The figure shows three views and two pictorial views of one solid part (mm, origin at its lowest corner). Answer the questions. Coordinates: 2 decimals unless noted, no trailing zeros. Loops run counter-clockwise (first coordinate to the right, second up) from the corner with the lowest first, then second, coordinate; pieces in that order, holes last. Notation, with made-up numbers: M 32.5,-3 L 85.5,-3 A14 ccw 85.5,11 Z; hole C -32,35.5 d8. An arc over 180 degrees is marked long. Return JSON: item names as keys, results as strings. Group by question number.
1. Given P1, Ø0.5, axis at x = 36.5, y = 36.5, coming from the +Z side; P2, Ø2.5, axis at x = 1, z = 16, coming from the -Y side; P3, Ø1.1, axis at x = 36, y = 36.5, coming from the -Z side; P4, Ø2.5, axis at x = 1, z = 16.5, coming from the -Y side, each flat-ended and moving along its own axis, determine where each tip first touches the part or whether it passes through.
2. Section B-B (z = 16.5) is taken. Write down the section's boundary in (x, y), then the cut area to 3 significant figures.
3. Section A-A (x = 19.25) is taken. Write down the section's boundary in (y, z), then the cut area to 3 significant figures.
4. Straight lines are drawn through the part: L1, parallel to Z at x = 1, y = 36.7; L2, parallel to X at y = 36.4, z = 16.5; L3, parallel to X at y = 26, z = 16.5. For each, find the intervals that lie inside material, in ascending order. Write a range as from..to.
5. Section D-D (x = 37.5) is taken. Write down the section's boundary in (y, z).
6. The mould has two halves that part along Z. Classify the marked faces 1, 2 and 3: pulls with the +Z half, pulls with the -Z half, needs draft (parallel to the pull), parting line crosses it, or undercut.
7. Section C-C (y = 3.5) is taken. Write down the section's boundary in (x, z).
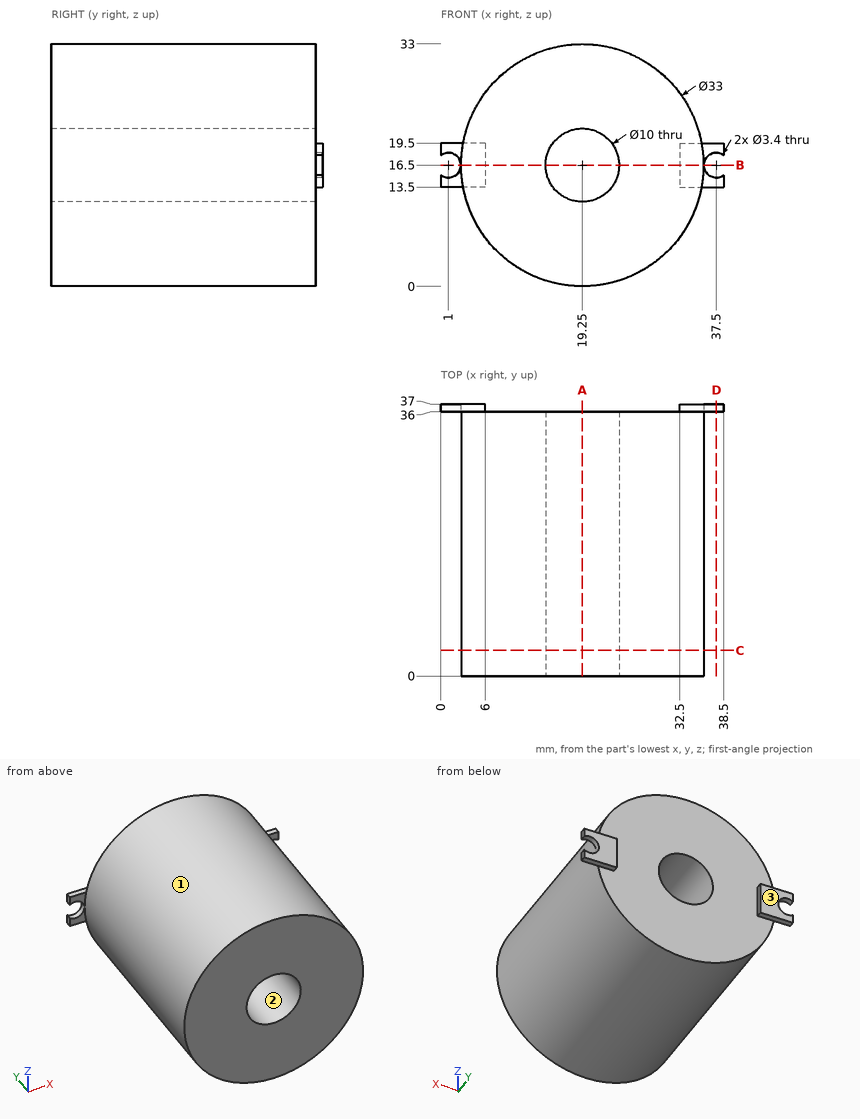
Worked out:
{
 "1": {"P1": "z = 19.5", "P2": "y = 36", "P3": "z = 13.5", "P4": "through"},
 "2": {"outline": "M 2.7,36 L 2.75,36 L 2.75,0 L 14.25,0 L 14.25,36 L 6,36 L 6,37 L 2.7,37 Z; M 24.25,0 L 35.75,0 L 35.75,36 L 35.8,36 L 35.8,37 L 32.5,37 L 32.5,36 L 24.25,36 Z", "area": "835 mm^2"},
 "3": {"outline": "M 0,0 L 36,0 L 36,11.5 L 0,11.5 Z; M 0,21.5 L 36,21.5 L 36,33 L 0,33 Z", "area": "828 mm^2"},
 "4": {"L1": "13.5..14.8, 18.2..19.5", "L2": "2.7..6, 32.5..35.8", "L3": "2.75..14.25, 24.25..35.75"},
 "5": {"outline": "M 36,13.5 L 37,13.5 L 37,14.8 L 36,14.8 Z; M 36,18.2 L 37,18.2 L 37,19.5 L 36,19.5 Z"},
 "6": {"face 1": "parting line crosses it", "face 2": "undercut", "face 3": "needs draft"},
 "7": {"outline": "C 19.25,16.5 d33; hole C 19.25,16.5 d10"}
}
